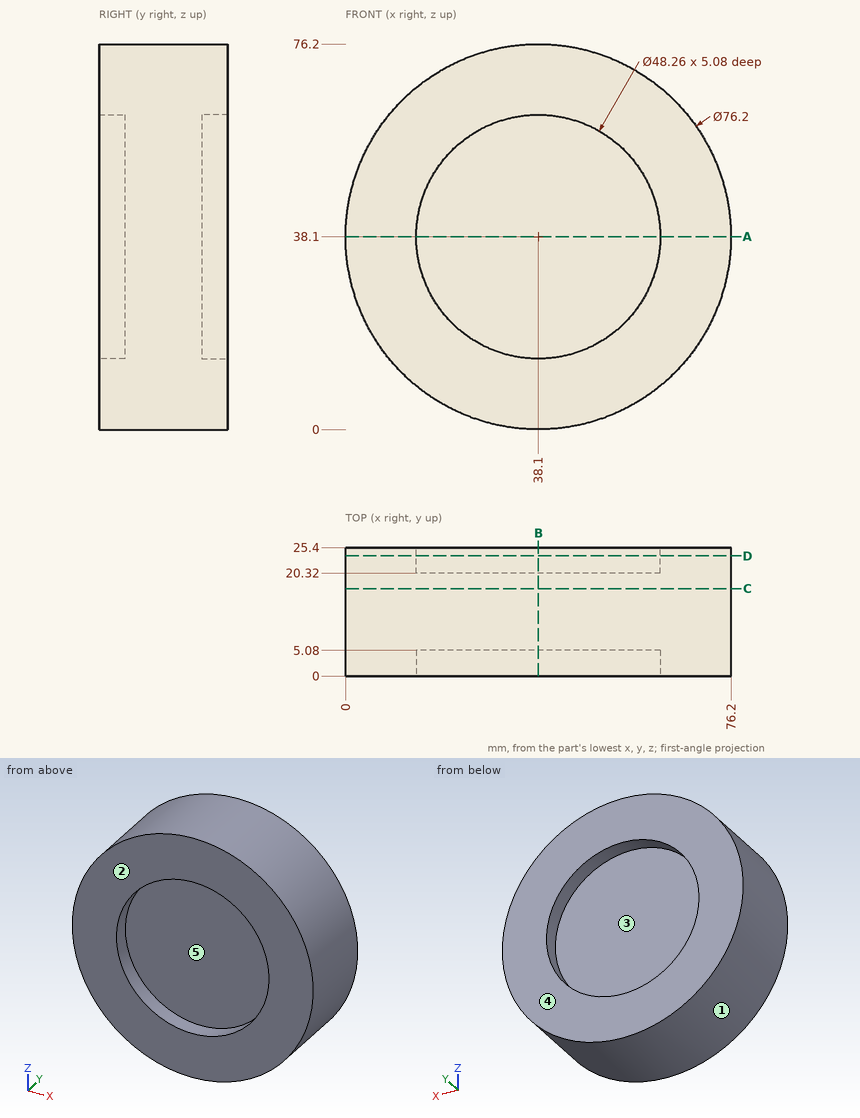
Design review of the part shown in the three views and the two pictorial views. Dimensions are in mm from the part's minimum x, y and z. A direction names the side the tool comes from. Round coordinates to 2 decimals unless told otherwise and drop trailing zeros. Write each loop counter-clockwise with the first axis right and the second up, starting at its lowest first coordinate (ties: lowest second). Pieces come first, ordered by that corner, then holes. Notation, with made-up numbers: (-28, -17.5) -> (15, -17.5) arc R10 ccw to (15, -9.5) -> close; hole circle Ø4 at (-7.5, 2). An arc over 180 degrees is marked (long way). One line per question, with ' | ' between items. Start each with the question number.
1) Add section A-A (z = 38.1). Write out the cut boundary in (x, y), and give its area (3 significant figures).
2) Machinability: for the marked faces 4 and 5, which of the approach directions +Z, -Z, +X, -X, +Y, -Y give a long, thin tool a straight path to every point of the face, cutting with its end or side? Answer none if there is none.
3) Add section B-B (x = 38.1). Write out the cut boundary in (y, z), and give its area (3 significant figures).
4) Mouldability with a two-part tool opening along X and no side actions: class the marked faces 1, 2 and 3 as +X half, -X half, draft (parallel to the pull), parting line (faces both ways), or undercut.
5) Wall thickness on line 1 along X through (y, z) = (1.9, 38.1); line 2 along Y through (x, z) = (26.5, 32.5); line 3 along Z through (x, y) = (18, 3.5): over which ranges is each line inside the solid? List them lowest first.
6) Add section D-D (y = 23.75). Write out the cut boundary in (x, z), and give its area (3 significant figures).
7) Add section C-C (y = 17.25). Write out the cut boundary in (x, z).
8) For pin 1 Ø5 at (y, z) = (6, 38) entering from -X; pin 2 Ø1.5 at (x, y) = (36, 20) entering from +Z; pin 3 Ø1 at (y, z) = (16, 67.5) entering from -X, all flat-tipped, find the tip position at first contact; note any pin that passes through.
Reported:
1) outline: (0, 0) -> (13.97, 0) -> (13.97, 5.08) -> (62.23, 5.08) -> (62.23, 0) -> (76.2, 0) -> (76.2, 25.4) -> (62.23, 25.4) -> (62.23, 20.32) -> (13.97, 20.32) -> (13.97, 25.4) -> (0, 25.4) -> close | area: 1,450 mm²
2) face 4: +Z, -Z, +X, -X, +Y | face 5: -Y
3) outline: (0, 0) -> (25.4, 0) -> (25.4, 13.97) -> (20.32, 13.97) -> (20.32, 62.23) -> (25.4, 62.23) -> (25.4, 76.2) -> (0, 76.2) -> (0, 62.23) -> (5.08, 62.23) -> (5.08, 13.97) -> (0, 13.97) -> close | area: 1,450 mm²
4) face 1: parting line | face 2: draft | face 3: undercut
5) line 1: x = 0 to 13.97, 62.23 to 76.2 | line 2: y = 5.08 to 20.32 | line 3: z = 5.73 to 24.75, 51.45 to 70.47
6) outline: circle Ø76.2 at (38.1, 38.1); hole circle Ø48.26 at (38.1, 38.1) | area: 2,730 mm²
7) outline: circle Ø76.2 at (38.1, 38.1)
8) pin 1: stops at x = 0 | pin 2: stops at z = 76.18 | pin 3: stops at x = 13.27
